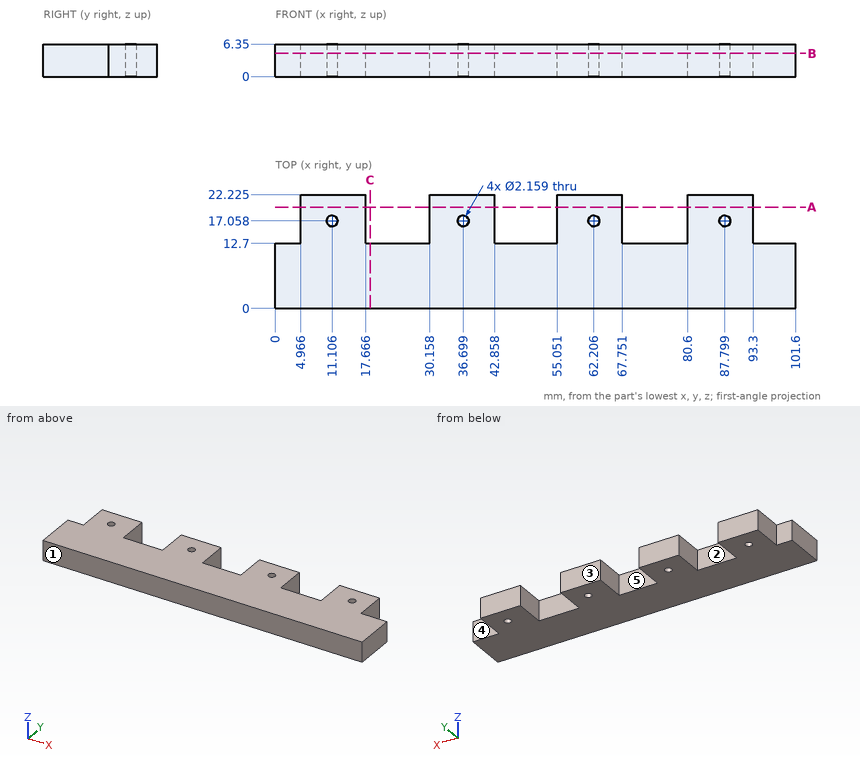
Could you check a few things on this drawing? It's one solid part, dimensions in mm from its lowest x, y, z. A direction names the side the tool comes from. Round coordinates to 2 decimals unless told otherwise and drop trailing zeros. Loops run counter-clockwise (first coordinate to the right, second up) from the corner with the lowest first, then second, coordinate; pieces in that order, holes last. Notation, with made-up numbers: (-6.5, 52.5) -> (48.5, 52.5) arc R25 cw to (48.5, 90.5) -> close; hole circle Ø11 at (54.25, 80.5). An arc over 180 degrees is marked (long way). Write each question's results on one line, items separated by ' | '.
(1) We'd pull the mould along X, two halves only. Please class the marked faces 1 and 2: released by +X, released by -X, zero draft, split by the parting line, or undercut.
Worked answers:
face 1: zero draft | face 2: undercut
(2) If I drill on L1, parallel to X at y = 21, z = 1.25; L2, parallel to Y at x = 88, z = 2 (1 decimal); L3, parallel to Y at x = 20, z = 0.5, over which ranges is the centre line in solid material (lowest first)?
Worked answers:
L1: 4.97 to 17.67, 30.16 to 42.86, 55.05 to 67.75, 80.6 to 93.3 | L2: 0 to 16, 18.1 to 22.2 | L3: 0 to 12.7
(3) If we section it at A-A, the plane y = 19.75: List the corners of the cut face in (x, z) for me.
Worked answers:
outline: (4.97, 0) -> (17.67, 0) -> (17.67, 6.35) -> (4.97, 6.35) -> close; (30.16, 0) -> (42.86, 0) -> (42.86, 6.35) -> (30.16, 6.35) -> close; (55.05, 0) -> (67.75, 0) -> (67.75, 6.35) -> (55.05, 6.35) -> close; (80.6, 0) -> (93.3, 0) -> (93.3, 6.35) -> (80.6, 6.35) -> close
(4) If we section it at B-B, the plane z = 4.5: List the corners of the cut face in (x, y) for me (1 decimal).
Worked answers:
outline: (0, 0) -> (101.6, 0) -> (101.6, 12.7) -> (93.3, 12.7) -> (93.3, 22.2) -> (80.6, 22.2) -> (80.6, 12.7) -> (67.8, 12.7) -> (67.8, 22.2) -> (55.1, 22.2) -> (55.1, 12.7) -> (42.9, 12.7) -> (42.9, 22.2) -> (30.2, 22.2) -> (30.2, 12.7) -> (17.7, 12.7) -> (17.7, 22.2) -> (5, 22.2) -> (5, 12.7) -> (0, 12.7) -> close; hole circle Ø2.2 at (11.1, 17.1); hole circle Ø2.2 at (36.7, 17.1); hole circle Ø2.2 at (62.2, 17.1); hole circle Ø2.2 at (87.8, 17.1)
(5) For the marked faces 3, 4 and 5, which set-ups out of +Z, -Z, +X, -X, +Y, -Y let a thin tool reach every point of the face, with its end or its side?
Worked answers:
face 3: +Z, -Z, +X, -X, +Y | face 4: +Z, -Z, +X, +Y | face 5: +Z, -Z, +Y
(6) For P1, Ø3, axis at y = 17.5, z = 3.5, coming from the -X side; P2, Ø3, axis at x = 36.7, y = 17.06, coming from the +Z side; P3, Ø3, axis at x = 47, z = 2.5, coming from the +Y side; P4, Ø3, axis at y = 18.5, z = 3, coming from the +X side, each with a flat end and sliding along its axis, tell me the tip position at first contact or that it passes through.
Worked answers:
P1: x = 4.97 | P2: z = 6.35 | P3: y = 12.7 | P4: x = 93.3
(7) If we section it at C-C, the plane x = 18.5: List the corners of the cut face in (y, z) for me.
Worked answers:
outline: (0, 0) -> (12.7, 0) -> (12.7, 6.35) -> (0, 6.35) -> close
